from build123d import *

# Parameters (mm, degrees)
PAD013_DEPTH            = 9
SKETCH034_R             = 11.25
POCKET003_DEPTH         = 7
SKETCH035_R             = 8
POCKET004_DEPTH         = 5
SKETCH040_W             = 16
SKETCH040_H             = 37
PAD016_DEPTH            = 24
SKETCH042_W             = 16
SKETCH042_H             = 7
PAD017_DEPTH            = 12
SKETCH043_W             = 12.5
SKETCH043_H             = 5.25
POCKET008_DEPTH         = 10
SKETCH044_R             = 1
POCKET009_DEPTH         = 4
POCKET009_DEPTH_BACK    = 5
SKETCH045_W             = 12.5
SKETCH045_H             = 25
POCKET010_DEPTH         = 50
SKETCH071_R             = 2.25
PAD027_DEPTH            = 14
SKETCH072_R             = 2.25
POCKET026_DEPTH         = 10
SKETCH073_W             = 16
SKETCH073_H             = 37
SKETCH073_W_2           = 14
SKETCH073_H_2           = 35
POCKET035_DEPTH         = 1
SKETCH084_W             = 10
SKETCH084_H             = 5
POCKET036_DEPTH         = 10
POCKET037_DEPTH         = 4
POCKET038_DEPTH         = 4
SKETCH133_W             = 12.5
SKETCH133_H             = 33
POCKET053_DEPTH         = 12
FILLET_R                = 2
BODY004_PLACEMENT_ANGLE = 90


with BuildPart() as part:
    # Sketch033 → Pad013 (new body)
    with BuildSketch(Plane.XY):
        with BuildLine():
            ThreePointArc((12.269609, 5), (-13.250782, 0), (12.269609, -5))
            Line((12.269609, -5), (47.729609, -5))
            ThreePointArc((47.729609, -5), (73.25, 0), (47.729609, 5))
            Line((12.269609, 5), (47.729609, 5))
        make_face()
    extrude(amount=PAD013_DEPTH)

    # Sketch034 (on Face6 of Pad013) → Pocket003 (cut)
    with BuildSketch(Plane.XY.offset(9)):
        Circle(SKETCH034_R)
        with Locations((60, 0)):
            Circle(SKETCH034_R)
    extrude(amount=-POCKET003_DEPTH, mode=Mode.SUBTRACT)

    # Sketch035 (on Face4 of Pocket003) → Pocket004 (cut)
    with BuildSketch(Plane(origin=(0, 0, 0), x_dir=(1, 0, 0), z_dir=(0, 0, -1))):
        Circle(SKETCH035_R)
        with Locations((60, 0)):
            Circle(SKETCH035_R)
    extrude(amount=-POCKET004_DEPTH, mode=Mode.SUBTRACT)

    # Sketch040 (on Face4 of Pocket004) → Pad016 (join)
    with BuildSketch(Plane(origin=(0, 0, 0), x_dir=(1, 0, 0), z_dir=(0, 0, -1))):
        with Locations((30, -4.5)):
            Rectangle(SKETCH040_W, SKETCH040_H)
    extrude(amount=-PAD016_DEPTH)

    # Sketch042 → Pad017 (join)
    with BuildSketch(Plane(origin=(0, 0, 0), x_dir=(1, 0, 0), z_dir=(0, 0, -1))):
        with Locations((30, -19.5)):
            Rectangle(SKETCH042_W, SKETCH042_H)
        with Locations((30, 10.5)):
            Rectangle(SKETCH042_W, SKETCH042_H)
    extrude(amount=-PAD017_DEPTH)

    # Sketch043 (on Face4 of Pad017) → Pocket008 (cut)
    with BuildSketch(Plane(origin=(0, 0, 0), x_dir=(1, 0, 0), z_dir=(0, 0, -1))):
        with Locations((30, 9.625)):
            Rectangle(SKETCH043_W, SKETCH043_H)
        with Locations((30, -18.625)):
            Rectangle(SKETCH043_W, SKETCH043_H)
    extrude(amount=-POCKET008_DEPTH, mode=Mode.SUBTRACT)

    # Sketch044 (on Face40 of Pocket008) → Pocket009 (cut, two sides)
    with BuildSketch(Plane(origin=(0, 0, 10), x_dir=(1, 0, 0), z_dir=(0, 0, -1))) as pocket009_sk:
        with Locations((30, -19)):
            Circle(SKETCH044_R)
        with Locations((30, 10)):
            Circle(SKETCH044_R)
    extrude(amount=-POCKET009_DEPTH, mode=Mode.SUBTRACT)
    extrude(pocket009_sk.sketch, amount=POCKET009_DEPTH_BACK, mode=Mode.SUBTRACT)

    # Sketch045 (on Face17 of Pocket009) → Pocket010 (cut)
    with BuildSketch(Plane(origin=(0, 0, 0), x_dir=(1, 0, 0), z_dir=(0, 0, -1))):
        with Locations((30, -4.5)):
            Rectangle(SKETCH045_W, SKETCH045_H)
    extrude(amount=-POCKET010_DEPTH, mode=Mode.SUBTRACT)

    # Sketch071 → Pad027 (join)
    with BuildSketch(Plane.XY.offset(9)):
        with BuildLine():
            ThreePointArc((43, -5), (48, 1e-05), (42.999979, 5))
            Line((37, 5), (42.999979, 5))
            Line((37, 5), (37, -5))
            Line((37, -5), (43, -5))
        make_face()
        with Locations((43, 0)):
            Circle(SKETCH071_R, mode=Mode.SUBTRACT)
        with BuildLine():
            ThreePointArc((17, 5), (12, 0), (17, -5))
            Line((23, -5), (17, -5))
            Line((23, 5), (23, -5))
            Line((17, 5), (23, 5))
        make_face()
        with Locations((17, 0)):
            Circle(SKETCH071_R, mode=Mode.SUBTRACT)
    extrude(amount=PAD027_DEPTH)

    # Sketch072 (on Face4 of Pad027) → Pocket026 (cut)
    with BuildSketch(Plane(origin=(0, 0, 0), x_dir=(1, 0, 0), z_dir=(0, 0, -1))):
        with Locations((17, 0)):
            Circle(SKETCH072_R)
        with Locations((43, 0)):
            Circle(SKETCH072_R)
    extrude(amount=-POCKET026_DEPTH, mode=Mode.SUBTRACT)

    # Sketch073 (on Face19 of Pocket026) → Pocket035 (cut)
    with BuildSketch(Plane.XY.offset(24)):
        with Locations((30, 4.5)):
            Rectangle(SKETCH073_W, SKETCH073_H)
        with Locations((30, 4.5)):
            Rectangle(SKETCH073_W_2, SKETCH073_H_2, mode=Mode.SUBTRACT)
    extrude(amount=-POCKET035_DEPTH, mode=Mode.SUBTRACT)

    # Sketch084 (on Face9 of Pocket035) → Pocket036 (cut)
    with BuildSketch(Plane.XZ.offset(5)):
        with Locations((17, 15.5)):
            Rectangle(SKETCH084_W, SKETCH084_H)
        with Locations((43, 15.5)):
            Rectangle(SKETCH084_W, SKETCH084_H)
    extrude(amount=-POCKET036_DEPTH, mode=Mode.SUBTRACT)

    # Sketch085 (on Face21 of Pocket036) → Pocket037 (cut)
    with BuildSketch(Plane.XY.offset(13)):
        Polygon((13, 0), (15, -3.464102), (19, -3.464102), (21, 0), (19, 3.464102), (15, 3.464102), align=None)
        Polygon((39, 0), (41, -3.464102), (45, -3.464102), (47, 0), (45, 3.464102), (41, 3.464102), align=None)
    extrude(amount=-POCKET037_DEPTH, mode=Mode.SUBTRACT)

    # Sketch086 (on Face30 of Pocket037) → Pocket038 (cut)
    with BuildSketch(Plane(origin=(0, 0, 18), x_dir=(1, 0, 0), z_dir=(0, 0, -1))):
        Polygon((13, 0), (15, -3.464102), (19, -3.464102), (21, 0), (19, 3.464102), (15, 3.464102), align=None)
        Polygon((39, 0), (41, -3.464102), (45, -3.464102), (47, 0), (45, 3.464102), (41, 3.464102), align=None)
    extrude(amount=-POCKET038_DEPTH, mode=Mode.SUBTRACT)

    # Sketch133 (on Face52 of Pocket038) → Pocket053 (cut)
    with BuildSketch(Plane.XY.offset(24)):
        with Locations((30, 4.5)):
            Rectangle(SKETCH133_W, SKETCH133_H)
    extrude(amount=-POCKET053_DEPTH, mode=Mode.SUBTRACT)

    # Fillet
    fillet_edges = [part.edges().sort_by_distance(p)[0] for p in [
        (38, -14, 6),
        (38, -14, 17.5),
        (22, -14, 17.5),
        (22, -14, 6),
        (22, 23, 17.5),
        (22, 23, 6),
        (38, 23, 6),
        (38, 23, 17.5),
    ]]
    fillet(fillet_edges, radius=FILLET_R)


with BuildPart() as part_1:
    # Body004 placement: moved
    add(part.part.moved(Location((0, 60, 0))).rotate(Axis((0, 60, 0), (0, 0, 1)), BODY004_PLACEMENT_ANGLE))


solid = part_1.part
Design review of the part built by this model. Coordinates are the model's own, in mm. A direction names the side the tool comes from. Round coordinates to 2 decimals unless told otherwise and drop trailing zeros. Write each loop counter-clockwise with the first axis right and the second up, starting at its lowest first coordinate (ties: lowest second). Pieces come first, ordered by that corner, then holes. Notation, with made-up numbers: (-21, 61) - (23, 61) arc R27 ccw to (23, 94) - close; hole circle Ø9 at (56, -1). An arc over 180 degrees is marked (long way). Use a Markdown table: item, result. Add a question column.
1. Wall thickness on probe 1 along Y at (x, z) = (-18.5, 16.25); probe 2 along X at (y, z) = (81.5, 5.75); probe 3 along Y at (x, z) = (-4, 22.75): over which ranges is each line inside the solid? List them lowest first.
2. Mouldability with a two-part tool opening along X and no side actions: class faces 5 (the face through (0, 108, 11)), 6 (the face through (14, 90, 11)), 7 (the face through (-1.708, 73.986, 19.972)), 8 (the face through (-1.756, 100.014, 11.028)) as +X half, -X half, draft (parallel to the pull), parting line (faces both ways), or undercut.
3. We need section A-A (y = 90). State the section outline as (x, z) points, then the cut area to 3 significant figures.
4. For faces 1 (the face through (-8, 122, 2)), 2 (the face through (5, 77, 5)), 3 (the face through (1.708, 99.986, 11.028)), 4 (the face through (-19.1, 88.5, 10)), list the 3-axis set-ups (+Z, -Z, +X, -X, +Y, -Y) from which the entire face can be reached by the end or side of a thin tool; tool diameter is ignored.
5. We need section B-B (x = -16). State the section outline as (y, z) points, then the cut area to 3 significant figures.
6. Clearance check with flat-ended pins moving along their axes: pin 1 (2 mm diameter, centred on x = -19, y = 92.5, fed in from -Z); pin 2 (3 mm diameter, centred on y = 103, z = 19.5, fed in from +X); pin 3 (5 mm diameter, centred on x = -15, y = 122.5, fed in from -Z); pin 4 (10 mm diameter, centred on y = 115, z = 10, fed in from -X). State where each tip first meets the part, or that it passes through.
7. We need section C-C (y = 60). State the section outline as (x, z) points, then the cut area to 3 significant figures.
8. We need section D-D (z = 16.5). State the section outline as (x, y) points.
Output:
| question | item | result |
|---|---|---|
| 1 | probe 1 | y = 82 to 83.75, 96.25 to 98 |
| 1 | probe 2 | x = -5 to 5 |
| 1 | probe 3 | y = 74 to 83.75, 96.25 to 106 |
| 2 | face 5 | parting line |
| 2 | face 6 | +X half |
| 2 | face 7 | undercut |
| 2 | face 8 | undercut |
| 3 | outline | (-23, 0) - (-21.25, 0) - (-21.25, 10) - (-20, 10) - (-20, 12) - (-21, 12) - (-21, 24) - (-22, 24) - (-22, 23) - (-23, 23) - close; (-18, 10) - (-17, 10) - (-17, 12) - (-18, 12) - close; (8, 10) - (9, 10) - (9, 12) - (8, 12) - close; (11, 10) - (12.25, 10) - (12.25, 0) - (14, 0) - (14, 23) - (13, 23) - (13, 24) - (12, 24) - (12, 12) - (11, 12) - close |
| 3 | area | 97.0 mm2 |
| 4 | face 1 | +Z |
| 4 | face 2 | +Z, -Z, +X |
| 4 | face 3 | none |
| 4 | face 4 | -Z |
| 5 | outline | (82, 0) - (83.75, 0) - (83.75, 24) - (83, 24) - (83, 23) - (82, 23) - close; (96.25, 0) - (98, 0) - (98, 23) - (97, 23) - (97, 24) - (96.25, 24) - close |
| 5 | area | 82.0 mm2 |
| 6 | pin 1 | stops at z = 10 |
| 6 | pin 2 | stops at x = 5 |
| 6 | pin 3 | stops at z = 0 |
| 6 | pin 4 | stops at x = -13.25 |
| 7 | outline | (-13.25, 0) - (-8, 0) - (-8, 2) - (-11.25, 2) - (-11.25, 9) - (-13.25, 9) - close; (8, 0) - (13.25, 0) - (13.25, 9) - (11.25, 9) - (11.25, 2) - (8, 2) - close |
| 7 | area | 49.0 mm2 |
| 8 | outline | (-23, 84) arc R2 ccw to (-21, 82) - (12, 82) arc R2 ccw to (14, 84) - (14, 96) arc R2 ccw to (12, 98) - (-21, 98) arc R2 ccw to (-23, 96) - close; hole (-21, 83.75) - (12, 83.75) - (12, 96.25) - (-21, 96.25) - close |
